Could you check a few things on this model? Use its own coordinates, in mm. Give positions to 0.01 mm unless a question says otherwise; leave off trailing zeros. Order: outer loops, then holes, each group sorted by start corner. A loop starts at its lowest first (then second) coordinate and runs counter-clockwise, first axis right, second up. Notation, with made-up numbers: M 47,84.25 L 88,84.25 A20 ccw 88,97.25 Z; hole C -7,39.25 d1. An arc over 180 degrees is marked long. Return JSON: item names as keys, results as strings. Group by question number.
```python
from build123d import *

# Parameters (mm, degrees)
BASE_DEPTH         = 6.35
SKETCH2_R          = 4.7752
SKETCH2_R_2        = 2.54
SKETCH2_R_3        = 3.96875
BOLTS_DEPTH        = 7.35
CUT_EXTRUDE1_DEPTH = 7.35


with BuildPart() as part:
    # Sketch1 → Base (new body)
    with BuildSketch(Plane(origin=(0, 0, 0), x_dir=(1, 0, 0), z_dir=(0, 1, 0))):
        with BuildLine():
            Line((-29.84179191, 198.076923077), (-49.736319849, 5.128205128))
            ThreePointArc((-49.736319849, 5.128205128), (-50, 0), (-49.736319849, -5.128205128))
            Line((-49.736319849, -5.128205128), (-29.84179191, -198.076923077))
            ThreePointArc((-29.84179191, -198.076923077), (0, -225), (29.84179191, -198.076923077))
            Line((29.84179191, -198.076923077), (49.736319849, -5.128205128))
            ThreePointArc((49.736319849, -5.128205128), (50, 0), (49.736319849, 5.128205128))
            Line((49.736319849, 5.128205128), (29.84179191, 198.076923077))
            ThreePointArc((29.84179191, 198.076923077), (0, 225), (-29.84179191, 198.076923077))
        make_face()
    extrude(amount=BASE_DEPTH)

    # Sketch2 → Bolts (cut, through all)
    with BuildSketch(Plane(origin=(0, 6.35, 0), x_dir=(1, 0, 0), z_dir=(0, 1, 0))):
        Circle(SKETCH2_R)
        with Locations((0, 195)):
            Circle(SKETCH2_R_2)
        with Locations((-23.8125, 0)):
            Circle(SKETCH2_R_3)
        with Locations((23.8125, 0)):
            Circle(SKETCH2_R_3)
        with Locations((0, -195)):
            Circle(SKETCH2_R_2)
    extrude(amount=-BOLTS_DEPTH, mode=Mode.SUBTRACT)

    # Sketch4 → Cut-Extrude1 (cut, through all)
    with BuildSketch(Plane(origin=(0, 6.35, 0), x_dir=(1, 0, 0), z_dir=(0, 1, 0))):
        with BuildLine():
            Line((-26.724762216, -33.307692308), (-24.340140182, -56.435145528))
            ThreePointArc((-24.340140182, -56.435145528), (-23.190453971, -60.163726372), (-20.701416296, -63.168520034))
            Line((-20.701416296, -63.168520034), (-6.308540083, -74.870782535))
            ThreePointArc((-6.308540083, -74.870782535), (0, -77.111767003), (6.308540083, -74.870782535))
            Line((6.308540083, -74.870782535), (20.701416296, -63.168520034))
            ThreePointArc((20.701416296, -63.168520034), (23.190453971, -60.163726372), (24.340140182, -56.435145528))
            Line((24.340140182, -56.435145528), (26.724762216, -33.307692308))
            ThreePointArc((26.724762216, -33.307692308), (25.968034139, -30.990407619), (23.740583026, -30))
            Line((23.740583026, -30), (-23.740583026, -30))
            ThreePointArc((-23.740583026, -30), (-25.968034139, -30.990407619), (-26.724762216, -33.307692308))
        make_face()
        with BuildLine():
            Line((16.120016428, -86.225819503), (7.759015532, -93.023809413))
            ThreePointArc((7.759015532, -93.023809413), (4.120291645, -99.757183919), (6.308540083, -107.091365027))
            Line((6.308540083, -107.091365027), (13.106529993, -115.452365924))
            ThreePointArc((13.106529993, -115.452365924), (16.291959962, -116.434574723), (18.418413843, -113.867496207))
            Line((18.418413843, -113.867496207), (20.996757644, -88.86121647))
            ThreePointArc((20.996757644, -88.86121647), (19.438845014, -85.914250835), (16.120016428, -86.225819503))
        make_face()
        with BuildLine():
            Line((-6.308540083, -107.091365027), (-13.106529993, -115.452365924))
            ThreePointArc((-13.106529993, -115.452365924), (-16.291959962, -116.434574723), (-18.418413843, -113.867496207))
            Line((-18.418413843, -113.867496207), (-20.996757644, -88.86121647))
            ThreePointArc((-20.996757644, -88.86121647), (-19.438845014, -85.914250835), (-16.120016428, -86.225819503))
            Line((-16.120016428, -86.225819503), (-7.759015532, -93.023809413))
            ThreePointArc((-7.759015532, -93.023809413), (-4.120291645, -99.757183919), (-6.308540083, -107.091365027))
        make_face()
        with BuildLine():
            Line((-7.759015532, -132.652629505), (-12.886782867, -138.95938604))
            ThreePointArc((-12.886782867, -138.95938604), (-14.710336749, -142.408841756), (-15.075031305, -146.293567149))
            Line((-15.075031305, -146.293567149), (-12.78933939, -168.461538462))
            ThreePointArc((-12.78933939, -168.461538462), (0, -180), (12.78933939, -168.461538462))
            Line((12.78933939, -168.461538462), (15.075031305, -146.293567149))
            ThreePointArc((15.075031305, -146.293567149), (14.710336749, -142.408841756), (12.886782867, -138.95938604))
            Line((12.886782867, -138.95938604), (7.759015532, -132.652629505))
            ThreePointArc((7.759015532, -132.652629505), (0, -128.961169588), (-7.759015532, -132.652629505))
        make_face()
        with BuildLine():
            Line((24.340140182, 56.435145528), (26.724762216, 33.307692308))
            ThreePointArc((26.724762216, 33.307692308), (25.968034139, 30.990407619), (23.740583026, 30))
            Line((23.740583026, 30), (-23.740583026, 30))
            ThreePointArc((-23.740583026, 30), (-25.968034139, 30.990407619), (-26.724762216, 33.307692308))
            Line((-26.724762216, 33.307692308), (-24.340140182, 56.435145528))
            ThreePointArc((-24.340140182, 56.435145528), (-23.190453971, 60.163726372), (-20.701416296, 63.168520034))
            Line((-20.701416296, 63.168520034), (-6.308540083, 74.870782535))
            ThreePointArc((-6.308540083, 74.870782535), (0, 77.111767003), (6.308540083, 74.870782535))
            Line((6.308540083, 74.870782535), (20.701416296, 63.168520034))
            ThreePointArc((20.701416296, 63.168520034), (23.190453971, 60.163726372), (24.340140182, 56.435145528))
        make_face()
        with BuildLine():
            Line((-16.120016428, 86.225819503), (-7.759015532, 93.023809413))
            ThreePointArc((-7.759015532, 93.023809413), (-4.120291645, 99.757183919), (-6.308540083, 107.091365027))
            Line((-6.308540083, 107.091365027), (-13.106529993, 115.452365924))
            ThreePointArc((-13.106529993, 115.452365924), (-16.291959962, 116.434574723), (-18.418413843, 113.867496207))
            Line((-18.418413843, 113.867496207), (-20.996757644, 88.86121647))
            ThreePointArc((-20.996757644, 88.86121647), (-19.438845014, 85.914250835), (-16.120016428, 86.225819503))
        make_face()
        with BuildLine():
            Line((6.308540083, 107.091365027), (13.106529993, 115.452365924))
            ThreePointArc((13.106529993, 115.452365924), (16.291959962, 116.434574723), (18.418413843, 113.867496207))
            Line((18.418413843, 113.867496207), (20.996757644, 88.86121647))
            ThreePointArc((20.996757644, 88.86121647), (19.438845014, 85.914250835), (16.120016428, 86.225819503))
            Line((16.120016428, 86.225819503), (7.759015532, 93.023809413))
            ThreePointArc((7.759015532, 93.023809413), (4.120291645, 99.757183919), (6.308540083, 107.091365027))
        make_face()
        with BuildLine():
            Line((12.78933939, 168.461538462), (15.075031305, 146.293567149))
            ThreePointArc((15.075031305, 146.293567149), (14.710336749, 142.408841756), (12.886782867, 138.95938604))
            Line((12.886782867, 138.95938604), (7.759015532, 132.652629505))
            ThreePointArc((7.759015532, 132.652629505), (0, 128.961169588), (-7.759015532, 132.652629505))
            Line((-7.759015532, 132.652629505), (-12.886782867, 138.95938604))
            ThreePointArc((-12.886782867, 138.95938604), (-14.710336749, 142.408841756), (-15.075031305, 146.293567149))
            Line((-15.075031305, 146.293567149), (-12.78933939, 168.461538462))
            ThreePointArc((-12.78933939, 168.461538462), (0, 180), (12.78933939, 168.461538462))
        make_face()
    extrude(amount=-CUT_EXTRUDE1_DEPTH, mode=Mode.SUBTRACT)


solid = part.part
```
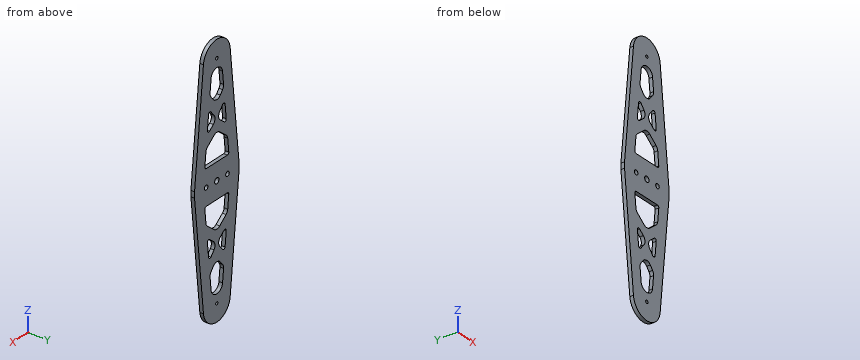
1. Imagine slicing it at B-B, the plane y = 4.75. Count the separate pieces of the cut face and the enclosed holes in it, plus the area to 3 significant figures.
2. For pin 1 (4.5 mm diameter, centred on x = 0, z = 195, fed in from -Y); pin 2 (2 mm diameter, centred on x = 16, y = 3, fed in from -Z); pin 3 (1.9 mm diameter, centred on x = -7, y = 4, fed in from -Z); pin 4 (3 mm diameter, centred on x = -6, y = 3, fed in from +Z), each with a flat end and sliding along its axis, tell me the tip position at first contact or that it passes through.
3. Imagine slicing it at A-A, the plane z = 0. Please give me the cut outline in (x, y).
4. I need wall thicknesses on L1, parallel to X at y = 1.5, z = 0; L2, parallel to Z at x = 16.5, y = 0.5; L3, parallel to Z at x = 3.5, y = 0.75. Which ranges of each line are inside material? Lowest first, please. Write a range as from..to.
Values:
{
 "1": {"separate pieces": "1", "enclosed holes": "13", "area": "26,100 mm²"},
 "2": {"pin 1": "passes through", "pin 2": "stops at z = -220.98", "pin 3": "stops at z = -224.38", "pin 4": "stops at z = 224.66"},
 "3": {"outline": "M -50,0 L -27.78,0 L -27.78,6.35 L -50,6.35 Z; M -19.84,0 L -4.78,0 L -4.78,6.35 L -19.84,6.35 Z; M 4.78,0 L 19.84,0 L 19.84,6.35 L 4.78,6.35 Z; M 27.78,0 L 50,0 L 50,6.35 L 27.78,6.35 Z"},
 "4": {"L1": "x = -50..-27.78, -19.84..-4.78, 4.78..19.84, 27.78..50", "L2": "z = -220.05..-116.36, -85.96..-66.58, -30..30, 66.58..85.96, 116.36..220.05", "L3": "z = -224.8..-179.51, -129.59..-76.48, -30..-3.25, 3.25..30, 76.48..129.59, 179.51..224.8"}
}
